```python
from build123d import *

# Parameters (mm, degrees)
F1_DEPTH  = 52.324
F3_DEPTH  = 26.925
F2_W      = 6.35
F2_H      = 17.526
F2_H_2    = 28.575
F2_H_3    = 11.049
F4_DEPTH  = 11.176
F6_DEPTH  = 26.925
F7_DEPTH  = 1.525
F8_W      = 69.596
F8_H      = 28.575
F9_DEPTH  = 6.35
F10_W     = 69.596
F10_H     = 28.575
F11_DEPTH = 6.35


with BuildPart() as f1:
    # F0 (on Right) → F1 (new body, symmetric)
    with BuildSketch(Plane.YZ):
        Polygon((-7.874, 26.924), (-7.874, 15.875), (7.874, 15.875), (7.874, 26.924), (12.7, 26.924), (12.7, 44.45), (-12.7, 44.45), (-12.7, 26.924), align=None)
        Polygon((-7.874, 15.875), (-14.224, 15.875), (-14.224, -15.875), (-7.874, -15.875), (7.874, -15.875), (14.224, -15.875), (14.224, 15.875), (7.874, 15.875), align=None)
        Polygon((7.874, -15.875), (-7.874, -15.875), (-7.874, -26.924), (-12.7, -26.924), (-12.7, -44.45), (12.7, -44.45), (12.7, -26.924), (7.874, -26.924), align=None)
    extrude(amount=F1_DEPTH, both=True)

    # F2 (on face) → F3 (cut, through all)
    with BuildSketch(Plane.XZ.offset(12.7)):
        with BuildLine():
            ThreePointArc((-22.098, 35.814), (-27.08184, 32.753268), (-26.606053, 26.924))
            Line((-26.606053, 26.924), (6.286053, 26.924))
            ThreePointArc((6.286053, 26.924), (6.76184, 32.753268), (1.778, 35.814))
            Line((1.778, 35.814), (-22.098, 35.814))
        make_face()
        with BuildLine():
            Line((6.286053, 26.924), (-26.606053, 26.924))
            ThreePointArc((-26.606053, 26.924), (-24.625268, 25.24216), (-22.098, 24.638))
            Line((-22.098, 24.638), (1.778, 24.638))
            ThreePointArc((1.778, 24.638), (4.305268, 25.24216), (6.286053, 26.924))
        make_face()
        with BuildLine():
            ThreePointArc((-22.098, -24.638), (-27.686, -30.226), (-22.098, -35.814))
            Line((-22.098, -35.814), (1.778, -35.814))
            ThreePointArc((1.778, -35.814), (7.366, -30.226), (1.778, -24.638))
            Line((1.778, -24.638), (-22.098, -24.638))
        make_face()
    extrude(amount=-F3_DEPTH, mode=Mode.SUBTRACT)

    # F2 (on face) → F4 (cut)
    with BuildSketch(Plane.XZ.offset(12.7)):
        with Locations((-49.149, 35.687)):
            Rectangle(F2_W, F2_H)
        with Locations((-49.149, -30.1625)):
            Rectangle(F2_W, F2_H_2)
        with Locations((-49.149, 21.3995)):
            Rectangle(F2_W, F2_H_3)
    extrude(amount=-F4_DEPTH, mode=Mode.SUBTRACT)

    # F5 (on face) → F6 (cut, through all)
    with BuildSketch(Plane.XZ.offset(12.7)):
        Polygon((52.324, -44.45), (52.324, 44.45), (23.749, 15.875), (19.939, 15.875), (19.939, 0), (19.939, -15.875), (23.749, -15.875), align=None)
    extrude(amount=-F6_DEPTH, mode=Mode.SUBTRACT)

    # F5 (on face) → F7 (cut, through all)
    with BuildSketch(Plane.XZ.offset(12.7)):
        Polygon((52.324, -44.45), (52.324, 44.45), (23.749, 15.875), (19.939, 15.875), (19.939, 0), (19.939, -15.875), (23.749, -15.875), align=None)
    extrude(amount=F7_DEPTH, mode=Mode.SUBTRACT)

    # F8 (on face) → F9 (cut)
    with BuildSketch(Plane.XZ.offset(14.224)):
        with Locations((-17.526, 30.1625)):
            Rectangle(F8_W, F8_H)
        with Locations((-17.526, -30.1625)):
            Rectangle(F8_W, F8_H)
    extrude(amount=-F9_DEPTH, mode=Mode.SUBTRACT)

    # F10 (on face) → F11 (cut)
    with BuildSketch(Plane(origin=(0, 14.224, 0), x_dir=(-1, 0, 0), z_dir=(0, 1, 0))):
        with Locations((17.526, 30.1625)):
            Rectangle(F10_W, F10_H)
        with Locations((17.526, -30.1625)):
            Rectangle(F10_W, F10_H)
    extrude(amount=-F11_DEPTH, mode=Mode.SUBTRACT)


solid = f1.part
```
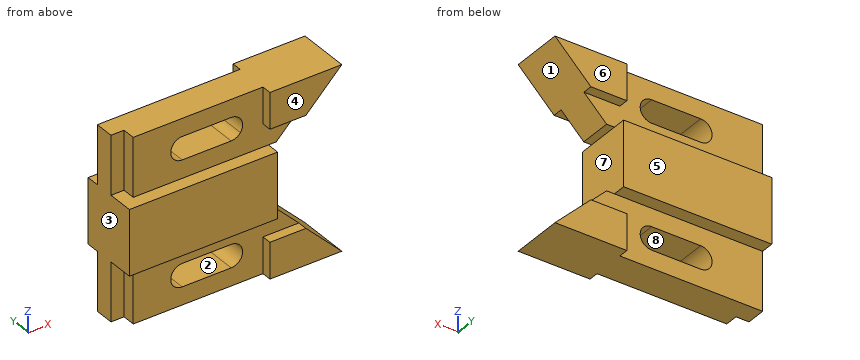
Check sheet for the modelled part. Datum: model origin and axes. Units: mm. Face numbers are marked on the shaded views. A direction names the side the tool comes from. Round coordinates to 2 decimals unless told otherwise and drop trailing zeros. Order: outer loops, then holes, each group sorted by start corner. A loop starts at its lowest first (then second) coordinate and runs counter-clockwise, first axis right, second up. Notation, with made-up numbers: (-20, -9.75) -> (13, -9.75) arc R30 ccw to (13, 20.25) -> close; hole circle Ø10 at (63, -8). An arc over 180 degrees is marked (long way). One line per item, written item: value. Start each with the question number.
Q1. Thickness scan on line 1 (Z direction, x = -10, y = -7); line 2 (Z direction, x = 22, y = -1.5) (3 decimals); line 3 (Z direction, x = 34, y = 10.25). Record the ranges inside material, lowest first.
Q2. Cross-section at C-C (y = -11.5). Record the boundary of the cut face in (x, z) (3 decimals), and give its area (3 significant figures).
Q3. Set-up check for the marked faces 5, 6, 7 and 8: record each of +Z, -Z, +X, -X, +Y, -Y from which the full face is reachable in a straight line by a thin tool's end or side.
Q4. Mould release check, pull along X, two halves, no side actions. Record for the marked faces 1, 2, 3 and 4: pulls with the +X half, pulls with the -X half, needs draft (parallel to the pull), parting line crosses it, or undercut.
Q5. Cross-section at A-A (y = 0.75). Record the boundary of the cut face in (x, z) (3 decimals).
Q6. Cross-section at D-D (z = 31). Record the boundary of the cut face in (x, y), and give its area (3 significant figures).
Q7. Cross-section at B-B (x = -9.5). Record the boundary of the cut face in (y, z) (3 decimals), and give its area (3 significant figures).
Q8. Gauge pin test, flat ends, axial feed: pin 1 Ø5 at (y, z) = (-4.5, -30) entering from -X; pin 2 Ø14.5 at (x, z) = (-5, -24) entering from -Y; pin 3 Ø12 at (y, z) = (-1.5, 19) entering from +X; pin 4 Ø6.5 at (x, y) = (-30, -9.5) entering from -Z. Record the tip position at first contact, or that the pin passes through.
Completed:
1. line 1: z = -44.45 to -35.81, -24.64 to 24.64, 35.81 to 44.45
1. line 2: z = -44.45 to -15.875, 15.875 to 44.45
1. line 3: z = -44.45 to -26.92, 26.92 to 44.45
2. outline: (-52.324, -15.875) -> (19.939, -15.875) -> (19.939, 15.875) -> (-52.324, 15.875) -> close; (17.272, -44.45) -> (52.324, -44.45) -> (34.798, -26.924) -> (17.272, -26.924) -> close; (17.272, 26.924) -> (34.798, 26.924) -> (52.324, 44.45) -> (17.272, 44.45) -> close
2. area: 3,220 mm²
3. face 5: +Z, -Z, +X, -X, +Y
3. face 6: +Z, +X, -X, +Y
3. face 7: +X, +Y, -Y
3. face 8: +Y, -Y
4. face 1: pulls with the +X half
4. face 2: undercut
4. face 3: pulls with the -X half
4. face 4: needs draft
5. outline: (-52.324, -44.45) -> (52.324, -44.45) -> (23.749, -15.875) -> (19.939, -15.875) -> (19.939, 15.875) -> (23.749, 15.875) -> (52.324, 44.45) -> (-52.324, 44.45) -> close; hole (-22.098, -35.814) -> (1.778, -35.814) arc R5.588 ccw to (1.778, -24.638) -> (-22.098, -24.638) arc R5.588 ccw to start; hole (-22.098, 24.638) -> (1.778, 24.638) arc R5.588 ccw to (1.778, 35.814) -> (-22.098, 35.814) arc R5.588 ccw to start
6. outline: (-52.32, -1.52) -> (-45.97, -1.52) -> (-45.97, -7.87) -> (-27.63, -7.87) -> (-27.63, 7.87) -> (-52.32, 7.87) -> close; (7.31, -7.87) -> (17.27, -7.87) -> (17.27, -12.7) -> (38.87, -12.7) -> (38.87, 12.7) -> (17.27, 12.7) -> (17.27, 7.87) -> (7.31, 7.87) -> close
6. area: 1,050 mm²
7. outline: (-14.224, -15.875) -> (-7.874, -15.875) -> (-7.874, -24.638) -> (7.874, -24.638) -> (7.874, -15.875) -> (14.224, -15.875) -> (14.224, 15.875) -> (7.874, 15.875) -> (7.874, 24.638) -> (-7.874, 24.638) -> (-7.874, 15.875) -> (-14.224, 15.875) -> close; (-7.874, -44.45) -> (7.874, -44.45) -> (7.874, -35.814) -> (-7.874, -35.814) -> close; (-7.874, 35.814) -> (7.874, 35.814) -> (7.874, 44.45) -> (-7.874, 44.45) -> close
7. area: 1,450 mm²
8. pin 1: stops at x = -45.97
8. pin 2: stops at y = -7.87
8. pin 3: stops at x = 32.87
8. pin 4: stops at z = -44.45
